from build123d import *

# Parameters (mm, degrees)
F0_R     = 58.1865618052
F1_DEPTH = 25.4
F1_TAPER = -3
F2_W     = 23.4757708386
F2_H     = 20.3105555847
F3_DEPTH = 25.4
F4_R     = 25.4
F5_W     = 30.9055270627
F5_H     = 11.7483213544
F6_DEPTH = 25.4


with BuildPart() as f1:
    # F0 (on Front) → F1 (new body)
    with BuildSketch(Plane.XZ):
        Circle(F0_R)
    extrude(amount=-F1_DEPTH, taper=F1_TAPER)

    # F2 (on face) → F3 (cut, through all)
    with BuildSketch(Plane.XZ):
        with Locations((-2.031555865, -0.8121863939)):
            Rectangle(F2_W, F2_H)
    extrude(amount=-F3_DEPTH, mode=Mode.SUBTRACT)

    # F4
    f4_edges = [f1.edges().sort_by_distance(p)[0] for p in [
        (-58.186562, 0, 0),
    ]]
    fillet(f4_edges, radius=F4_R)

    # F5 (on face) → F6 (join)
    with BuildSketch(Plane(origin=(0, 25.4, 0), x_dir=(-1, 0, 0), z_dir=(0, 1, 0))):
        with Locations((-19.417067524, 33.8719151914)):
            Rectangle(F5_W, F5_H)
    extrude(amount=F6_DEPTH)


solid = f1.part
Part model, mm, in its own coordinate system. A direction names the side the tool comes from. Coordinates: 2 decimals unless noted, no trailing zeros. Order: outer loops, then holes, each group sorted by start corner. A loop starts at its lowest first (then second) coordinate and runs counter-clockwise, first axis right, second up.
(1) Pin check, flat tips, straight feed: pin 1 Ø12 at (x, y) = (6.5, 17.5) entering from -Z; pin 2 Ø8 at (x, y) = (-34.5, 33) entering from +Z; pin 3 Ø10 at (y, z) = (13, 3) entering from +X; pin 4 Ø6 at (x, z) = (40.5, 11) entering from -Y. Stop position of each tip, or through.
Check sheet entries:
pin 1: stops at z = -59.24
pin 2: passes through
pin 3: stops at x = 58.32
pin 4: stops at y = 0.47
(2) Slice it at B-B, the plane y = 27. Write the cut outline in (x, z).
Check sheet entries:
outline: (3.96, 28) - (34.87, 28) - (34.87, 39.75) - (3.96, 39.75) - close
(3) Slice it at A-A, the plane x = 0. Write the cut outline in (y, z), and give its area (3 significant figures).
Check sheet entries:
outline: (0, -34.08) arc R25.4 ccw to (24.07, -59.45) - (25.4, -59.52) - (25.4, -10.97) - (0, -10.97) - close; (0, 9.34) - (25.4, 9.34) - (25.4, 59.52) - (24.07, 59.45) arc R25.4 ccw to (0, 34.08) - close
area: 2,230 mm2
(4) Tool access for faces 5 (the face through (20, 50.8, 34)), 6 (the face through (20, 38, 27.998)), 7 (the face through (-2, 13, -10.967)): list every direction of +Z, -Z, +X, -X, +Y, -Y with a clear straight run to the whole face (end or side of a thin tool).
Check sheet entries:
face 5: +Z, -Z, +X, -X, +Y
face 6: -Z, +X, -X, +Y
face 7: +Y, -Y
(5) Probe L1, parallel to Y at x = -29.5, z = 4; L2, parallel to X at y = 3, z = 6; L3, parallel to X at y = 25, z = -8.5. List the from-to ranges inside material, lowest first.
Check sheet entries:
L1: y = 0 to 25.4
L2: x = -45.67 to -13.77, 9.71 to 45.67
L3: x = -58.89 to -13.77, 9.71 to 58.89
(6) Pull direction X, two halves, no side cores. Call faces 1 (the face through (34.87, 38, 34)), 2 (the face through (-2, 13, 9.343)), 3 (the face through (20, 38, 39.746)), 4 (the face through (3.964, 38, 34)): pulls with the +X half, pulls with the -X half, needs draft (parallel to the pull), parting line crosses it, or undercut.
Check sheet entries:
face 1: pulls with the +X half
face 2: undercut
face 3: needs draft
face 4: pulls with the -X half
